Study the drawing (mm; zero at the part's minimum x, y, z) and answer. A direction names the side the tool comes from. Coordinates: 2 decimals unless noted, no trailing zeros. Order: outer loops, then holes, each group sorted by start corner. A loop starts at its lowest first (then second) coordinate and runs counter-clockwise, first axis right, second up. Notation, with made-up numbers: (81, 13.5) -> (113, 13.5) arc R18 cw to (113, 48.5) -> close; hole circle Ø2 at (7, -40). An arc over 180 degrees is marked (long way). Answer as CSV lines item,"result". Start each with the question number.
Item 1: Section B-B (y = 2.5) is taken. Write down the section's boundary in (x, z).
Item 2: Section A-A (x = 5) is taken. Write down the section's boundary in (y, z), then the cut area to 4 significant figures.
Item 3: Section C-C (z = 8.75) is taken. Write down the section's boundary in (x, y).
Item 4: Straight lines are drawn through the part: L1, parallel to Z at x = 3.15, y = 0.5; L2, parallel to X at y = 3.25, z = 6.75; L3, parallel to Y at x = 4.6, z = 0.5. For each, find the intervals that lie inside material, in ascending order.
Item 5: Each of these flat-tipped pins is pushed along its axis until it touches: pin 1 Ø1 at (x, y) = (2.5, 5.5) entering from -Z; pin 2 Ø0.6 at (x, y) = (2.5, 6.5) entering from +Z; pin 3 Ø1.2 at (y, z) = (5, 5) entering from +X. Where does it stop, or does it pass through?
Item 6: For a pull along Z with two mould halves and no side action, classify the marked faces 5, 6, 7 and 8 as pulls with the +Z half, pulls with the -Z half, needs draft (parallel to the pull), parting line crosses it, or undercut.
Item 7: Section D-D (y = 0.75) is taken. Write down the section's boundary in (x, z) (3 decimals).
Item 8: Which of the six approach directions +Z, -Z, +X, -X, +Y, -Y give full straight-line access (tool end or side, diameter ignored) to the marked faces 1, 2, 3 and 4?
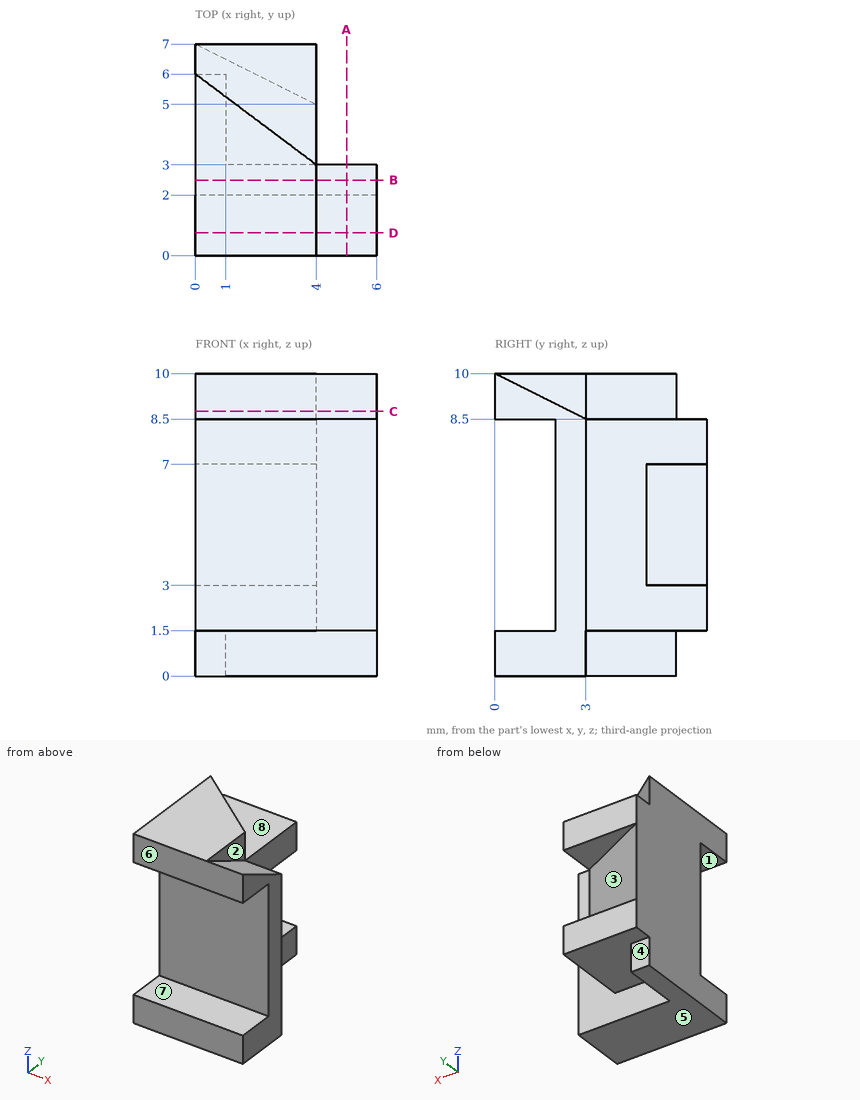
Checked values:
1,outline,"(0, 0) -> (6, 0) -> (6, 8.75) -> (4, 8.75) -> (4, 10) -> (0, 10) -> close"
2,outline,"(0, 0) -> (3, 0) -> (3, 8.5) -> (0, 10) -> (0, 8.5) -> (2, 8.5) -> (2, 1.5) -> (0, 1.5) -> close"
2,area,"13.75 mm^2"
3,outline,"(0, 0) -> (6, 0) -> (6, 2.5) -> (4, 2.5) -> (4, 3) -> (0, 6) -> close"
4,L1,"z = 0 to 1.5, 8.5 to 10"
4,L2,"x = 0 to 4"
4,L3,"y = 0 to 3"
5,pin 1,"stops at z = 1.5"
5,pin 2,"stops at z = 8.5"
5,pin 3,"stops at x = 4"
6,face 5,"pulls with the -Z half"
6,face 6,"needs draft"
6,face 7,"undercut"
6,face 8,"pulls with the +Z half"
7,outline,"(0, 0) -> (6, 0) -> (6, 1.5) -> (0, 1.5) -> close; (0, 8.5) -> (6, 8.5) -> (6, 9.625) -> (4, 9.625) -> (4, 10) -> (0, 10) -> close"
8,face 1,"+X, -X, -Y"
8,face 2,"+Z, +X, +Y"
8,face 3,"+X, +Y"
8,face 4,"-Z, +X, -X, +Y"
